Here's the drawing with two shaded views (mm, measured from the low corner). I have some questions. A direction names the side the tool comes from. Coordinates: 2 decimals unless noted, no trailing zeros. Order: outer loops, then holes, each group sorted by start corner. A loop starts at its lowest first (then second) coordinate and runs counter-clockwise, first axis right, second up. Notation, with made-up numbers: (-5, 88.25) -> (49, 88.25) arc R18 cw to (49, 111.25) -> close; hole circle Ø6 at (9, 40.25). An arc over 180 degrees is marked (long way). Return JSON: item names as keys, results as strings. Group by question number.
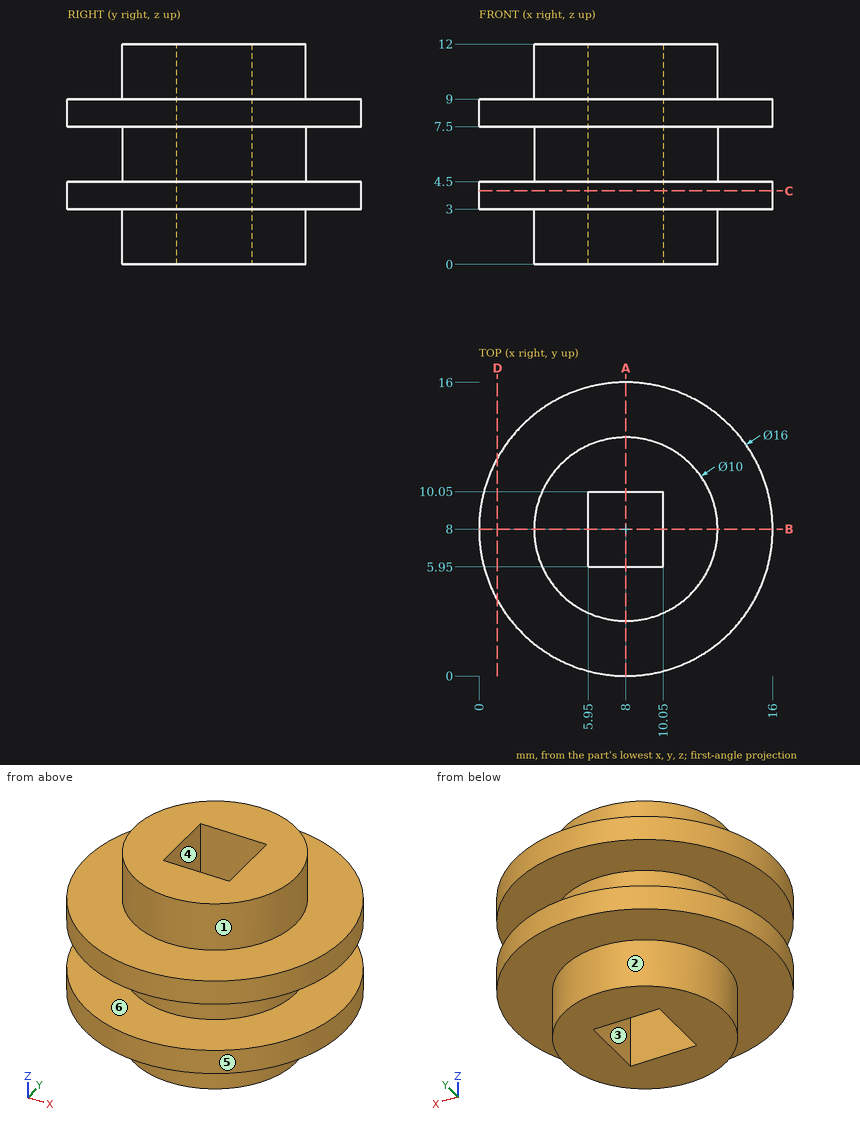
Q1. I want a section at D-D on x = 1. Please give me the cut outline in (y, z), and give its area (3 significant figures).
Q2. I want a section at A-A on x = 8. Please give me the cut outline in (y, z), and give its area (3 significant figures).
Q3. We'd pull the mould along X, two halves only. Please class the marked faces 4, 5 and 6: pulls with the +X half, pulls with the -X half, needs draft (parallel to the pull), parting line crosses it, or undercut.
Q4. I need wall thicknesses on line 1 along Y through (x, z) = (8.25, 7.75); line 2 along Z through (x, y) = (11.75, 14.25); line 3 along X through (y, z) = (6.5, 10.25). Which ranges of each line are inside material? Lowest first, please. Write a range as from..to.
Q5. I want a section at C-C on z = 4. Please give me the cut outline in (x, y), and give its area (3 significant figures).
Q6. I'm going to push flat-ended pins straight in: pin 1 Ø4 at (y, z) = (3.5, 3) entering from -X; pin 2 Ø4 at (y, z) = (5.5, 3.5) entering from -X; pin 3 Ø1 at (x, z) = (12, 4.5) entering from -Y. Where does each tip first touch, or does it pass through?
Q7. On a 3-axis mill with a long thin cutter (end or side, diameter ignored), from which of +Z, -Z, +X, -X, +Y, -Y can I reach the whole of each face in a straight line? I mean the marked faces 1, 2 and 3. Say none if no direction works.
Response values:
{
 "1": {"outline": "(4.13, 3) -> (11.87, 3) -> (11.87, 4.5) -> (4.13, 4.5) -> close; (4.13, 7.5) -> (11.87, 7.5) -> (11.87, 9) -> (4.13, 9) -> close", "area": "23.2 mm²"},
 "2": {"outline": "(0, 3) -> (3, 3) -> (3, 0) -> (5.95, 0) -> (5.95, 12) -> (3, 12) -> (3, 9) -> (0, 9) -> (0, 7.5) -> (3, 7.5) -> (3, 4.5) -> (0, 4.5) -> close; (10.05, 0) -> (13, 0) -> (13, 3) -> (16, 3) -> (16, 4.5) -> (13, 4.5) -> (13, 7.5) -> (16, 7.5) -> (16, 9) -> (13, 9) -> (13, 12) -> (10.05, 12) -> close", "area": "88.8 mm²"},
 "3": {"face 4": "undercut", "face 5": "parting line crosses it", "face 6": "needs draft"},
 "4": {"line 1": "y = 0..5.95, 10.05..16", "line 2": "z = 3..4.5, 7.5..9", "line 3": "x = 3.23..5.95, 10.05..12.77"},
 "5": {"outline": "circle Ø16 at (8, 8); hole (5.95, 5.95) -> (10.05, 5.95) -> (10.05, 10.05) -> (5.95, 10.05) -> close", "area": "184 mm²"},
 "6": {"pin 1": "stops at x = 0.4", "pin 2": "stops at x = 0.02", "pin 3": "stops at y = 0.81"},
 "7": {"face 1": "+Z", "face 2": "-Z", "face 3": "+Z, -Z"}
}
